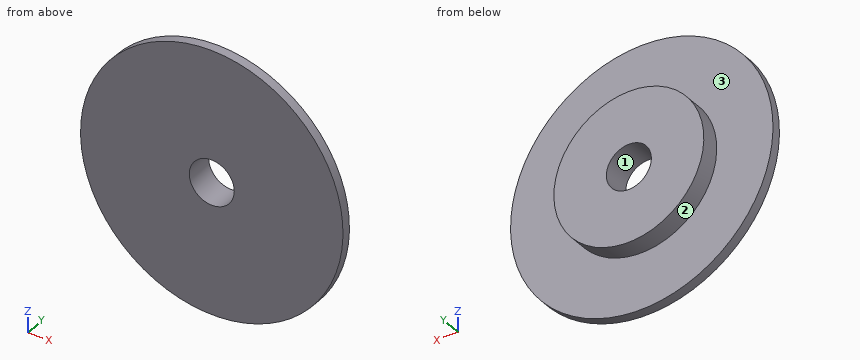
from build123d import *

# Parameters (mm, degrees)
SKETCH1_R                = 7
BOSS_EXTRUDE1_DEPTH      = 1.5
CUT_EXTRUDE1_START       = -1
SKETCH2_R                = 7
SKETCH2_R_2              = 4
CUT_EXTRUDE1_DEPTH       = 1
M2_CLEARANCE_HOLE1_D     = 2.4
M2_CLEARANCE_HOLE1_DEPTH = 3
M2_CLEARANCE_HOLE1_TIP   = 0.721032743


with BuildPart() as part:
    # Sketch1 → Boss-Extrude1 (new body)
    with BuildSketch(Plane(origin=(0, 0, 0), x_dir=(1, 0, 0), z_dir=(0, 1, 0))):
        with Locations(Location((0, 0, 0), (0, 0, 270))):
            Circle(SKETCH1_R)
    extrude(amount=BOSS_EXTRUDE1_DEPTH)

    # Sketch2 → Cut-Extrude1 (cut)
    with BuildSketch(Plane(origin=(0, 1.5, 0), x_dir=(1, 0, 0), z_dir=(0, 1, 0)).offset(CUT_EXTRUDE1_START)):
        with Locations(Location((0, 0, 0), (0, 0, 270))):
            Circle(SKETCH2_R)
        with Locations(Location((0, 0, 0), (0, 0, 270))):
            Circle(SKETCH2_R_2, mode=Mode.SUBTRACT)
    extrude(amount=CUT_EXTRUDE1_DEPTH, mode=Mode.SUBTRACT)

    # M2 Clearance Hole1
    with Locations(Plane(origin=(0, 0, 0), x_dir=(-1, 0, 0), z_dir=(0, -1, 0))):
        with Locations((0, 0)):
            Hole(M2_CLEARANCE_HOLE1_D / 2, depth=M2_CLEARANCE_HOLE1_DEPTH)
            with Locations((0, 0, -(M2_CLEARANCE_HOLE1_DEPTH + M2_CLEARANCE_HOLE1_TIP / 2))):  # 118° drill point
                Cone(0, M2_CLEARANCE_HOLE1_D / 2, M2_CLEARANCE_HOLE1_TIP, mode=Mode.SUBTRACT)


solid = part.part
Can you work these out from the model? Positions are in its coordinate system, mm. Face numbers are marked on the shaded views. Coordinates: 2 decimals unless noted, no trailing zeros. Order: outer loops, then holes, each group sorted by start corner. A loop starts at its lowest first (then second) coordinate and runs counter-clockwise, first axis right, second up. Notation, with made-up numbers: (84.25, -30) - (134.25, -30) arc R31 ccw to (134.25, 7) - close; hole circle Ø5 at (19, 60.5). An arc over 180 degrees is marked (long way). Answer as a JSON object with one key per item and string values. Group by question number.
Q1. Imagine slicing it at B-B (x = 0). Please give me the cut outline in (y, z).
Q2. Imagine slicing it at C-C (z = -1.5). Please give me the cut outline in (x, y).
Q3. I need wall thicknesses on line 1 (Y direction, x = -4, z = 0.5); line 2 (X direction, y = 0.45, z = 0.75); line 3 (Z direction, x = -1, y = 0.1). Which ranges of each line are inside material? Lowest first, please. Write a range as from..to.
Q4. Imagine slicing it at D-D (y = 0.8). Please give me the cut outline in (x, z).
Q5. Imagine slicing it at A-A (z = 0). Please give me the cut outline in (x, y), and give its area (3 significant figures).
Q6. We'd pull the mould along Z, two halves only. Please class the marked faces 1, 2 and 3: +Z half, -Z half, draft (parallel to the pull), parting line (faces both ways), or undercut.
Determined:
{
 "1": {"outline": "(0, -7) - (0.5, -7) - (0.5, -4) - (1.5, -4) - (1.5, -1.2) - (0, -1.2) - close; (0, 1.2) - (1.5, 1.2) - (1.5, 4) - (0.5, 4) - (0.5, 7) - (0, 7) - close"},
 "2": {"outline": "(-6.84, 0) - (6.84, 0) - (6.84, 0.5) - (3.71, 0.5) - (3.71, 1.5) - (-3.71, 1.5) - (-3.71, 0.5) - (-6.84, 0.5) - close"},
 "3": {"line 1": "y = 0..0.5", "line 2": "x = -6.96..-0.94, 0.94..6.96", "line 3": "z = -6.93..-0.66, 0.66..6.93"},
 "4": {"outline": "circle Ø8 at (0, 0); hole circle Ø2.4 at (0, 0)"},
 "5": {"outline": "(-7, 0) - (-1.2, 0) - (-1.2, 1.5) - (-4, 1.5) - (-4, 0.5) - (-7, 0.5) - close; (1.2, 0) - (7, 0) - (7, 0.5) - (4, 0.5) - (4, 1.5) - (1.2, 1.5) - close", "area": "11.4 mm2"},
 "6": {"face 1": "undercut", "face 2": "parting line", "face 3": "draft"}
}
